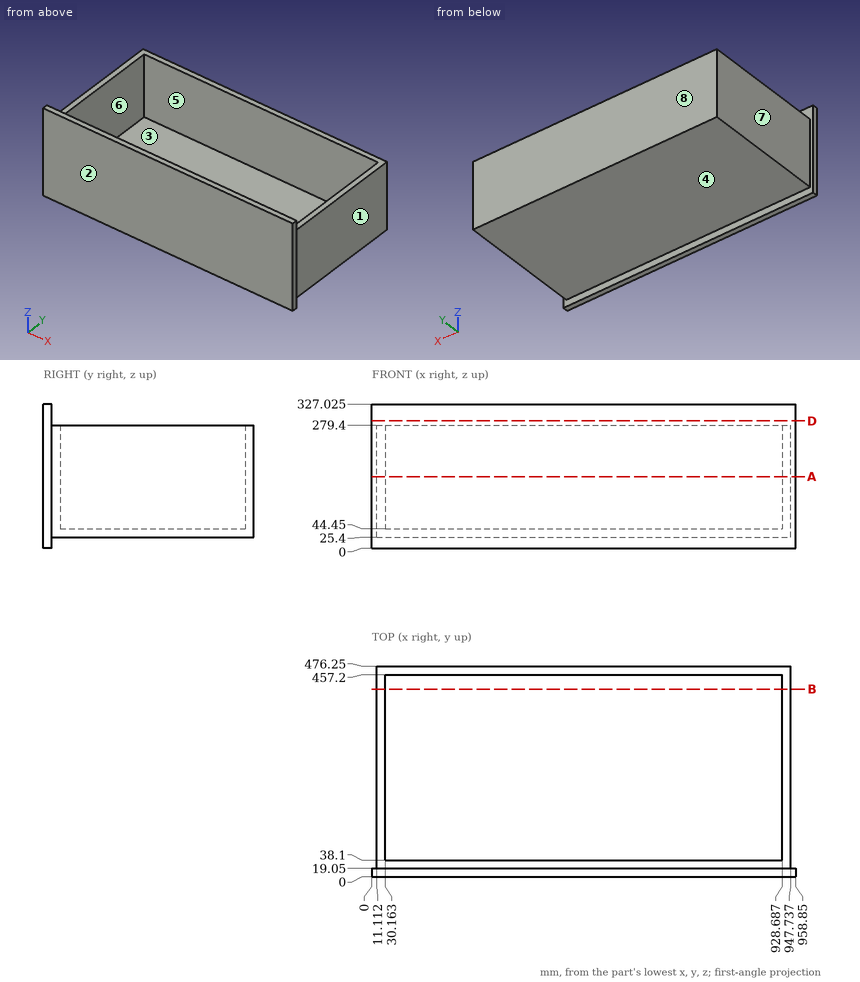
Could you check a few things on this drawing? It's one solid part, dimensions in mm from its lowest x, y, z. A direction names the side the tool comes from. Give positions to 0.01 mm unless a question says otherwise; leave off trailing zeros. Order: outer loops, then holes, each group sorted by start corner. A loop starts at its lowest first (then second) coordinate and runs counter-clockwise, first axis right, second up.
1. Which directions (+Z, -Z, +X, -X, +Y, -Y) give clear straight access to the entire face, cutting with the end or side of a thin tool? Please do the marked faces 1, 2, 3 and 4.
Answers below:
face 1: +Z, -Z, +X, +Y
face 2: +Z, -Z, +X, -X, -Y
face 3: +Z
face 4: -Z, +X, -X, +Y
2. Suppose I cut it at D-D (z = 289). Write out the boundary of the cut face in (x, y).
Answers below:
outline: (0, 0) - (958.85, 0) - (958.85, 19.05) - (0, 19.05) - close
3. I need wall thicknesses on L1, parallel to X at y = 354, z = 267.5; L2, parallel to Y at x = 592.5, z = 249.5; L3, parallel to Z at x = 496.5, y = 324. Which ranges of each line are inside material? Lowest first, please.
Answers below:
L1: x = 11.11 to 30.16, 928.69 to 947.74
L2: y = 0 to 38.1, 457.2 to 476.25
L3: z = 25.4 to 44.45
4. Thinking about a two-plate mould opening in X: for the marked faces 5, 6, 7 and 8, which applies, +X half, -X half, draft (parallel to the pull), parting line (faces both ways), or undercut?
Answers below:
face 5: undercut
face 6: undercut
face 7: -X half
face 8: draft
5. For pin 1 (2 mm diameter, centred on y = 74.5, z = 232, fed in from +X); pin 2 (3 mm diameter, centred on x = 673, y = 48, fed in from +Z); pin 3 (1 mm diameter, centred on x = 829, y = 136.5, fed in from -Z), each with a flat end and sliding along its axis, tell me the tip position at first contact or that it passes through.
Answers below:
pin 1: stops at x = 947.74
pin 2: stops at z = 44.45
pin 3: stops at z = 25.4
6. Suppose I cut it at B-B (y = 425). Write out the boundary of the cut face in (x, z).
Answers below:
outline: (11.11, 25.4) - (947.74, 25.4) - (947.74, 279.4) - (928.69, 279.4) - (928.69, 44.45) - (30.16, 44.45) - (30.16, 279.4) - (11.11, 279.4) - close
7. Suppose I cut it at A-A (z = 162.5). Write out the boundary of the cut face in (x, y).
Answers below:
outline: (0, 0) - (958.85, 0) - (958.85, 19.05) - (947.74, 19.05) - (947.74, 476.25) - (11.11, 476.25) - (11.11, 19.05) - (0, 19.05) - close; hole (30.16, 38.1) - (928.69, 38.1) - (928.69, 457.2) - (30.16, 457.2) - close
